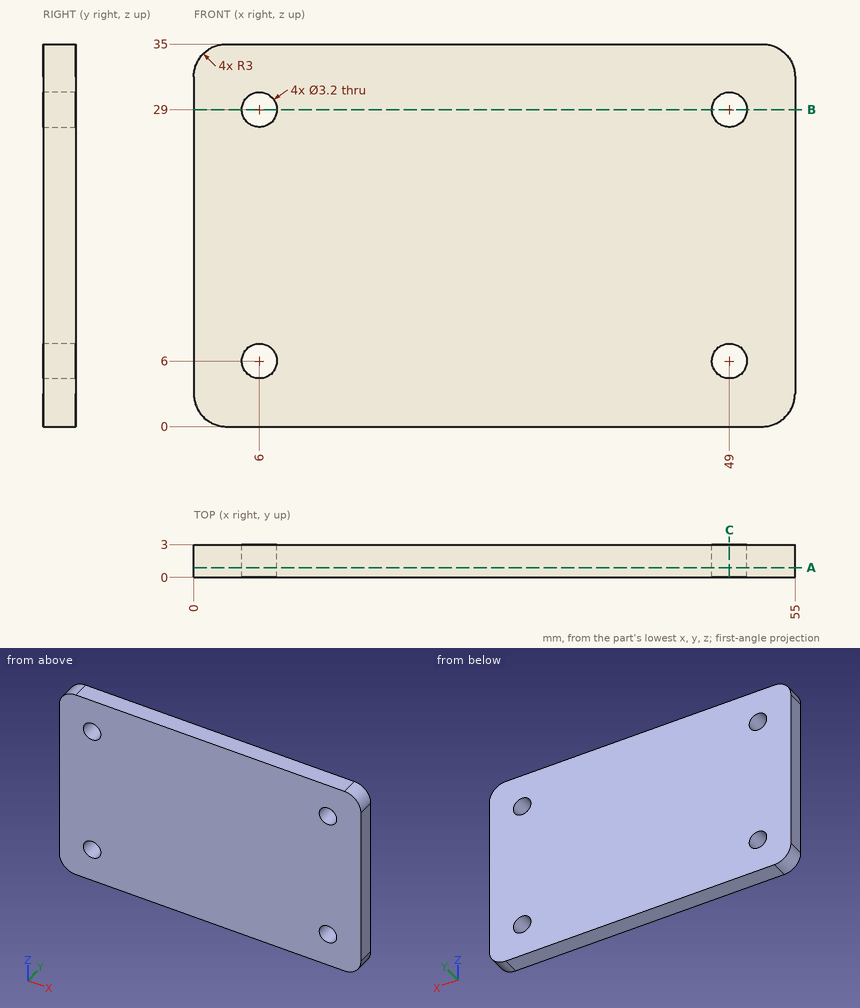
The figure shows three views and two pictorial views of one solid part (mm, origin at its lowest corner). Answer the questions. Round coordinates to 2 decimals unless told otherwise and drop trailing zeros. Write each loop counter-clockwise with the first axis right and the second up, starting at its lowest first coordinate (ties: lowest second). Pieces come first, ordered by that corner, then holes. Notation, with made-up numbers: (59.5, 55.25) -> (99.5, 55.25) arc R26 cw to (99.5, 89.25) -> close; hole circle Ø8 at (-28.5, 56.25). An arc over 180 degrees is marked (long way). Answer as a JSON object with one key per item and string values. Group by question number.
Q1. Section B-B (z = 29) is taken. Write down the section's boundary in (x, y), plus the area to 3 significant figures.
Q2. Section C-C (x = 49) is taken. Write down the section's boundary in (y, z).
Q3. This flat-tipped pin is pushed along its axis until it touches: pin 1 Ø1.9 at (x, z) = (6, 6) entering from -Y. Where does it stop, or does it pass through?
Q4. Section A-A (y = 0.9) is taken. Write down the section's boundary in (x, z), plus the area to 3 significant figures.
Q5. Straight lines are drawn through the part: line 1 along X through (y, z) = (1.8, 29); line 2 along X through (y, z) = (2, 6.5); line 3 along Z through (x, y) = (48, 2.5). For each, find the intervals that lie inside material, in ascending order.
Check values:
{
 "1": {"outline": "(0, 0) -> (4.4, 0) -> (4.4, 3) -> (0, 3) -> close; (7.6, 0) -> (47.4, 0) -> (47.4, 3) -> (7.6, 3) -> close; (50.6, 0) -> (55, 0) -> (55, 3) -> (50.6, 3) -> close", "area": "146 mm^2"},
 "2": {"outline": "(0, 0) -> (3, 0) -> (3, 4.4) -> (0, 4.4) -> close; (0, 7.6) -> (3, 7.6) -> (3, 27.4) -> (0, 27.4) -> close; (0, 30.6) -> (3, 30.6) -> (3, 35) -> (0, 35) -> close"},
 "3": {"pin 1": "through"},
 "4": {"outline": "(0, 3) arc R3 ccw to (3, 0) -> (52, 0) arc R3 ccw to (55, 3) -> (55, 32) arc R3 ccw to (52, 35) -> (3, 35) arc R3 ccw to (0, 32) -> close; hole circle Ø3.2 at (6, 6); hole circle Ø3.2 at (6, 29); hole circle Ø3.2 at (49, 6); hole circle Ø3.2 at (49, 29)", "area": "1,890 mm^2"},
 "5": {"line 1": "0 to 4.4, 7.6 to 47.4, 50.6 to 55", "line 2": "0 to 4.48, 7.52 to 47.48, 50.52 to 55", "line 3": "0 to 4.75, 7.25 to 27.75, 30.25 to 35"}
}
